Check sheet for the modelled part. Datum: model origin and axes. Units: mm. Face numbers are marked on the shaded views. A direction names the side the tool comes from. Round coordinates to 2 decimals unless told otherwise and drop trailing zeros. Loops run counter-clockwise (first coordinate to the right, second up) from the corner with the lowest first, then second, coordinate; pieces in that order, holes last. Notation, with made-up numbers: M -13.5,59 L 21.5,59 A30 ccw 21.5,94 Z; hole C -2.5,87 d1. An arc over 180 degrees is marked long. One line per question, with ' | ' between items. Start each with the question number.
(1) Thickness scan on probe 1 along X at (y, z) = (-1.25, 7.5); probe 2 along Y at (x, z) = (11.25, -4); probe 3 along Y at (x, z) = (4.25, -1). Record the ranges inside material, lowest first. Write a range as [from, to].
(2) Section check A-A (z = -3.25). Record the boundary of the cut face in (x, y).
(3) Tool access check on the marked faces 4 and 5. Record the directions out of +Z, -Z, +X, -X, +Y, -Y that give a thin tool (end or side, any length) a straight path to the whole face; none if there is none.
(4) Go/stop test with flat-tipped pins: P1, Ø0.8, axis at x = 0.5, z = -1.5, coming from the +Y side; P2, Ø1, axis at y = -2.5, z = 0.5, coming from the -X side. Record where each tip stops, or that it passes through.
(5) Section check D-D (y = -5). Record the boundary of the cut face in (x, z), and give its area (3 significant figures).
(6) Draft check along Z on the marked faces 1, 2 and 3. Enter one of: +Z half, -Z half, draft (parallel to the pull), parting line (faces both ways), or undercut.
(7) Section check B-B (y = 7.25). Record the boundary of the cut face in (x, z), and give its area (3 significant figures).
(8) Section check C-C (x = 11.25). Record the boundary of the cut face in (y, z).
Autodesk Inventor part; units mm, degrees
ref_plane "YZ Plane" through (0, 0, 0) normal (1, 0, 0) x (0, 1, 0)
ref_plane "XZ Plane" through (0, 0, 0) normal (0, 1, 0) x (-1, 0, 0)
ref_plane "XY Plane" through (0, 0, 0) normal (0, 0, 1) x (1, 0, 0)
sketch "Sketch1" plane through (0, 0, 0) normal (1, 0, 0) x (0, 1, 0)
  line L0 (10.5655, 7.5) -> (-10.5655, 7.5)
  line L1 (-10.5655, 7.5) -> (-10.5655, -6.983)
  line L2 (-10.5655, -6.983) -> (10.5655, -6.983)
  line L3 (10.5655, -6.983) -> (10.5655, 7.5)
  point P0 (0, 0)
  dimension "d0" = 21.131
  dimension "d2" = 10.5655
  dimension "d3" = 7.5
  dimension "d27" = 14.483
extrude "Extrusion1" add sketch "Sketch1" along normal blind 9
sketch "Sketch3" plane through (9, 0, 0) normal (1, 0, 0) x (0, 0, -1)
  circle A0 centre (3.983, 6.2605) radius 1.5
  point P0 (0, 0)
  dimension "d12" = 3
extrude "Extrusion3" add sketch "Sketch3" along normal blind 3
sketch "Sketch4" plane through (0, 0, 0) normal (-1, 0, 0) x (0, 0, 1)
  line L0 (-2.5186, -3.6831) -> (10.3419, -3.6831) construction
  line L1 (10.3419, -3.6831) -> (10.3419, -8.8157) construction
  line L2 (10.3419, -8.8157) -> (-2.5186, -8.8157) construction
  line L3 (-2.5186, -8.8157) -> (-2.5186, -3.6831) construction
  line L4 (-0.5697, -6.741) -> (-2.0567, -6.741)
  line L5 (-2.0567, -6.741) -> (-2.0567, -6.4297)
  line L6 (-2.0567, -6.4297) -> (-1.5034, -6.4297)
  line L7 (-1.5034, -6.4297) -> (-1.5034, -4.387)
  line L8 (-1.5034, -4.387) -> (-2.0567, -4.387)
  line L9 (-2.0567, -4.387) -> (-2.0567, -4.1079)
  spline S0 degree 2 poles (-2.0567, -4.1079) (-1.743, -4.1079) (-1.4466, -3.9301) (-1.4268, -3.6831) knots 0 0 0 1 2 2 2
  line L10 (-1.4268, -3.6831) -> (-1.1106, -3.6831)
  line L11 (-1.1106, -3.6831) -> (-1.1106, -6.4297)
  line L12 (-1.1106, -6.4297) -> (-0.5697, -6.4297)
  line L13 (-0.5697, -6.4297) -> (-0.5697, -6.741)
  line L14 (-0.2511, -6.741) -> (0.7764, -3.693)
  line L15 (0.7764, -3.693) -> (1.2754, -3.693)
  line L16 (1.2754, -3.693) -> (2.3029, -6.741)
  line L17 (2.3029, -6.741) -> (1.8756, -6.741)
  line L18 (1.8756, -6.741) -> (1.599, -5.8888)
  line L19 (1.599, -5.8888) -> (0.4356, -5.8888)
  line L20 (0.4356, -5.8888) -> (0.1589, -6.741)
  line L21 (0.1589, -6.741) -> (-0.2511, -6.741)
  line L22 (1.4878, -5.543) -> (1.016, -4.1079)
  line L23 (1.016, -4.1079) -> (0.5467, -5.543)
  line L24 (0.5467, -5.543) -> (1.4878, -5.543)
  point P0 (0, 0)
emboss "Emboss1" sketch "Sketch4" operation cut depth 1 direction (1, 0, 0)
sketch "Sketch6" plane through (0, -10.5655, -6.983) normal (0, -1, 0) x (1, 0, 0)
  line L0 (0, 14.483) -> (0, 0)
  line L1 (9, 14.483) -> (9, 0)
  line L2 (0, 0) -> (9, 0)
  line L3 (9, 0) -> (9, 14.483)
  line L4 (9, 14.483) -> (0, 14.483)
  line L5 (0, 14.483) -> (0, 0)
  point P0 (0, 6.983)
extrude "Extrusion5" add sketch "Sketch6" along normal blind 0.174
sketch "Sketch7" plane through (0, 10.5655, 7.5) normal (0, 0, 1) x (1, 0, 0)
  line L0 (0, 0) -> (9, 0)
  line L1 (9, 0) -> (9, -21.305)
  line L2 (0, 0) -> (9, 0)
  line L3 (9, 0) -> (9, -21.305)
  line L4 (9, -21.305) -> (0, -21.305)
  line L5 (0, -21.305) -> (0, 0)
  point P0 (0, -10.5655)
extrude "Extrusion6" add sketch "Sketch7" along normal blind 0.517
sketch "Sketch10" plane through (0, 10.5655, 8.017) normal (0, 1, 0) x (1, 0, 0)
  line L0 (0, 15) -> (9, 15)
  line L1 (9, 15) -> (9, 0)
  line L2 (0, 15) -> (9, 15)
  line L3 (9, 15) -> (9, 0)
  line L4 (9, 0) -> (0, 0)
  line L5 (0, 0) -> (0, 15)
  point P0 (0, 8.017)
  point P1 (9, 8.019)
  point P2 (9, 8.019)
extrude "Extrusion9" cut sketch "Sketch10" against normal blind 1.302
sketch "Sketch11" plane through (0, 0, 0) normal (-1, 0, 0) x (0, 0, 1)
  circle A0 centre (-1.502, 9.3028) radius 1.5
  line L0 (8.017, 9.2635) -> (8.017, -10.7395)
  point P0 (0, 0)
  dimension "d40" = 3
  dimension "d41" = 9.519
extrude "Extrusion10" cut sketch "Sketch11" against normal up to surface (9 mm away)
properties part number "Support_1A"
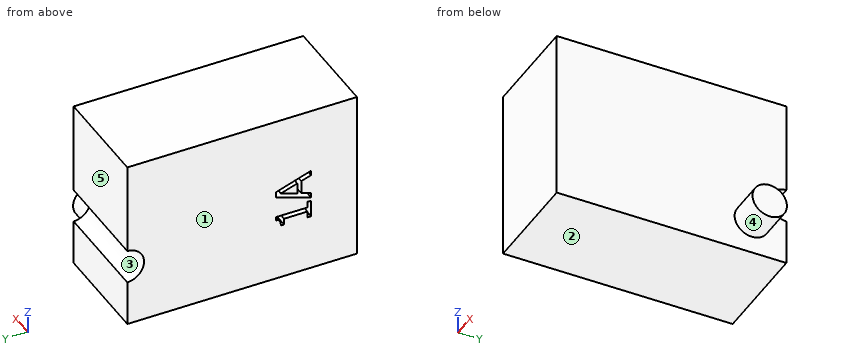
The answers:
1) probe 1: [0, 9] | probe 2: [4.76, 7.76] | probe 3: [-10.74, 7.89]
2) outline: M 0,-10.74 L 9,-10.74 L 9,4.95 L 12,4.95 L 12,7.57 L 9,7.57 L 9,9.26 L 0,9.26 Z
3) face 4: +X | face 5: +Z, -Z, +X, -X, +Y
4) P1: y = 7.86 | P2: x = 0
5) outline: M 0,-6.98 L 9,-6.98 L 9,8.02 L 0,8.02 L 0,1.72 L 1,1.72 L 1,1.31 L 0,1.31 L 0,0.72 L 1,0.72 L 1,0.34 L 0,0.34 L 0,-1.11 L 1,-1.11 L 1,-1.5 L 0,-1.5 Z | area: 134 mm²
6) face 1: draft | face 2: -Z half | face 3: undercut
7) outline: M 0,-6.98 L 9,-6.98 L 9,-5.11 L 12,-5.11 L 12,-2.86 L 9,-2.86 L 9,8.02 L 0,8.02 Z | area: 142 mm²
8) outline: C 6.26,-3.98 d3
